Here's the drawing with two shaded views (mm, measured from the low corner). I have some questions. Coordinates: 2 decimals unless noted, no trailing zeros. Write each loop counter-clockwise with the first axis right and the second up, starting at its lowest first coordinate (ties: lowest second). Pieces come first, ordered by that corner, then holes. Notation, with made-up numbers: M 10,31.5 L 34,31.5 A21 cw 34,64.5 Z; hole C 80,23 d5. An arc over 180 degrees is marked long. Use one line per item in the form item = value. Start each with the question number.
1. I want a section at A-A, the plane z = 17.5. List the corners of the cut face in (x, y) for me.
2. I want a section at C-C, the plane y = 5. List the corners of the cut face in (x, z) for me.
3. I'm going to push a flat-ended pin straight in: pin 1 Ø12 at (x, z) = (17.5, 17.5) entering from -Y. Where does the tip first touch, or does it pass through?
4. I want a section at B-B, the plane x = 17.5. List the corners of the cut face in (y, z) for me, plus the area to 3 significant figures.
5. Please list where these lines run through material, in increasing order: line 1 along X through (y, z) = (4.75, 17.5); line 2 along Z through (x, y) = (14.5, 3.75). Write a range as [from, to].
6. Thinking about a two-plate mould opening in X: for the marked faces 1, 2 and 3, which applies, released by +X, released by -X, zero draft, split by the parting line, or undercut?
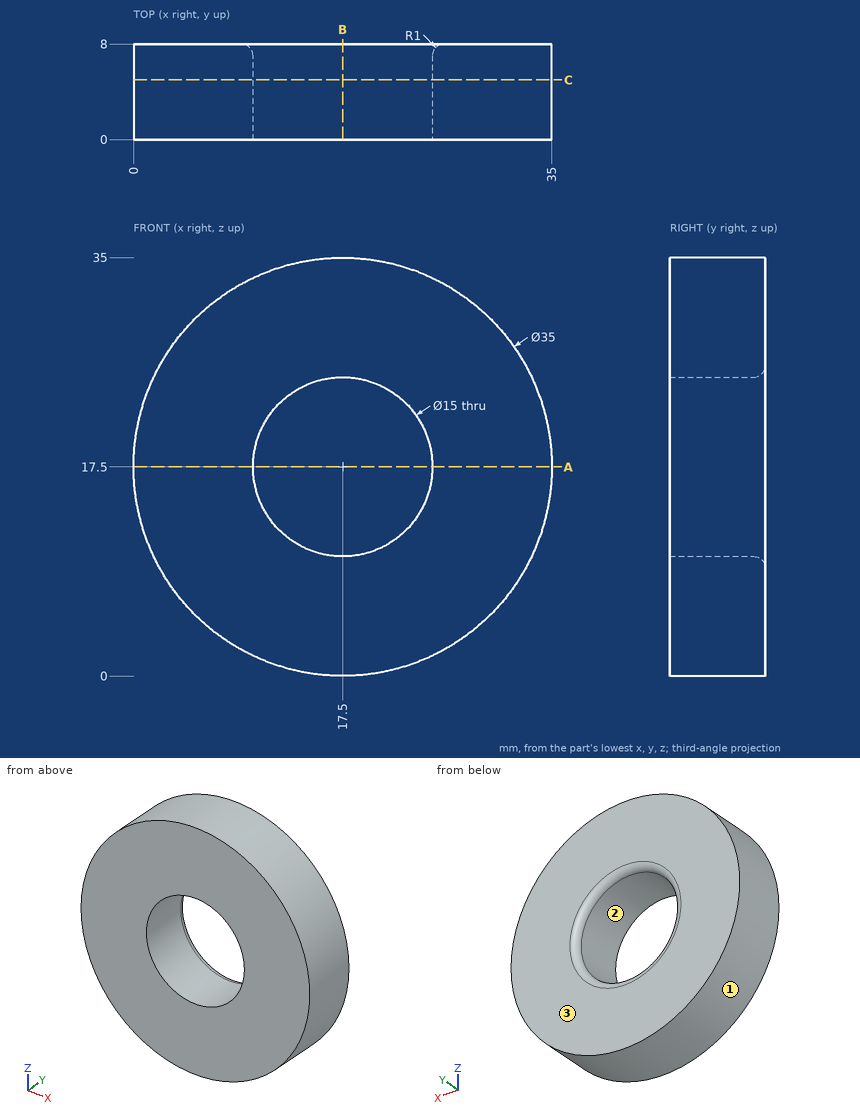
Answer list:
q1.outline = M 0,0 L 10,0 L 10,7 A1 ccw 9,8 L 0,8 Z; M 25,0 L 35,0 L 35,8 L 26,8 A1 ccw 25,7 Z
q2.outline = C 17.5,17.5 d35; hole C 17.5,17.5 d15
q3.pin_1 = through
q4.outline = M 0,0 L 8,0 L 8,9 A1 ccw 7,10 L 0,10 Z; M 0,25 L 7,25 A1 ccw 8,26 L 8,35 L 0,35 Z
q4.area = 160 mm²
q5.line_1 = [0, 10], [25, 35]
q5.line_2 = [0.26, 10.63], [24.37, 34.74]
q6.face_1 = split by the parting line
q6.face_2 = undercut
q6.face_3 = zero draft
